```python
from build123d import *

# Parameters (mm, degrees)
F0_W     = 73.5
F0_H     = 5
F1_DEPTH = 10
F2_W     = 68.2
F2_H     = 5
F3_DEPTH = 8
F4_R     = 4
F5_DEPTH = 2
F6_W     = 5
F6_H     = 2
F7_DEPTH = 76.5
F8_R     = 3.99999
F9_DEPTH = 2.5
F10_R    = 4


# Not quite as in the source:
# - a fillet or chamfer is up to 0.001 mm smaller than in the source, because OpenCascade refuses the exact size


with BuildPart() as f1:
    # F0 (on Top) → F1 (new body)
    with BuildSketch(Plane.XY):
        Rectangle(F0_W, F0_H)
    extrude(amount=F1_DEPTH)

    # F2 (on face) → F3 (cut)
    with BuildSketch(Plane.XY.offset(10)):
        Rectangle(F2_W, F2_H)
    extrude(amount=-F3_DEPTH, mode=Mode.SUBTRACT)

    # F4
    f4_edges = [f1.edges().sort_by_distance(p)[0] for p in [
        (34.1, 0, 2),
        (-34.1, 0, 2),
    ]]
    fillet(f4_edges, radius=F4_R)

    # F5 (add): a face of the model
    f5_faces = [f1.faces().sort_by_distance(p)[0] for p in [
        (-35.425, 0, 10),
    ]]
    extrude(f5_faces, amount=F5_DEPTH)

    # F6 (on face) → F7 (join)
    with BuildSketch(Plane.YZ.offset(-34.1)):
        with Locations((0, 11)):
            Rectangle(F6_W, F6_H)
    extrude(amount=F7_DEPTH)

    # F8 (radius 4 in the source; OpenCascade refuses exactly that, so slightly less here)
    f8_edges = [f1.edges().sort_by_distance(p)[0] for p in [
        (-34.1, 0, 10),
        (34.1, 0, 10),
    ]]
    fillet(f8_edges, radius=F8_R)

    # F9 (cut): a face of the model
    f9_faces = [f1.faces().sort_by_distance(p)[0] for p in [
        (2.825, 0, 12),
    ]]
    extrude(f9_faces, amount=-F9_DEPTH, mode=Mode.SUBTRACT)

    # F10
    f10_edges = [f1.edges().sort_by_distance(p)[0] for p in [
        (36.75, 0, 0),
        (-36.75, 0, 9.5),
        (-36.75, 0, 0),
        (36.75, 0, 9.5),
    ]]
    fillet(f10_edges, radius=F10_R)


solid = f1.part
```
Input: part model. Units: mm. Frame: model coordinates. A direction names the side the tool comes from. Coordinates: 2 decimals unless noted, no trailing zeros. Loops run counter-clockwise (first coordinate to the right, second up) from the corner with the lowest first, then second, coordinate; pieces in that order, holes last. Notation, with made-up numbers: (-11, 81) -> (38, 81) arc R12 ccw to (38, 86) -> close; hole circle Ø5 at (39, 51). An arc over 180 degrees is marked (long way). Use a Markdown table: item, result.
1) Cut plane A-A (z = 8.25). Return the cut outline in (x, y), then the cut area to 3 significant figures.
Results found:
| item | result |
|---|---|
| outline | (-35.65, -2.5) -> (-33.41, -2.5) -> (-33.41, 2.5) -> (-35.65, 2.5) -> close; (33.41, -2.5) -> (35.65, -2.5) -> (35.65, 2.5) -> (33.41, 2.5) -> close |
| area | 22.5 mm2 |
2) Access query for faces 1 (the cylindrical face through (32.959, 0.035, 3.203)), 2 (the cylindrical face through (-35.547, 0.035, 1.141)), 3 (the flat face through (0, 0, 2)). Directions: +Z, -Z, +X, -X, +Y, -Y. A direction counts if a zero-diameter tool reaches every point of the face in a straight line with its end or side. Return the directions, or none.
Results found:
| item | result |
|---|---|
| face 1 | +Y, -Y |
| face 2 | -Z, -X, +Y, -Y |
| face 3 | +Z, +Y, -Y |
3) Cut plane C-C (x = 21.5). Return the cut outline in (y, z), then the cut area to 3 significant figures.
Results found:
| item | result |
|---|---|
| outline | (-2.5, 0) -> (2.5, 0) -> (2.5, 2) -> (-2.5, 2) -> close |
| area | 10.0 mm2 |
4) Pull-direction query (Z, two-part tool) for faces 4 (the flat face through (0, 0, 0)), 5 (the cylindrical face through (33.56, 0.04, 8.01)), 6 (the flat face through (-36.75, 0, 5)); classes: released by +Z, released by -Z, zero draft, split by the parting line, or undercut.
Results found:
| item | result |
|---|---|
| face 4 | released by -Z |
| face 5 | undercut |
| face 6 | zero draft |
5) Material intervals for line 1 along Z through (x, y) = (29, -1.35); line 2 along X through (y, z) = (0.9, 4); line 3 along Z through (x, y) = (-32.5, -2.2), sorted ascending. Write a range as from..to.
Results found:
| item | result |
|---|---|
| line 1 | z = 0..2 |
| line 2 | x = -36.75..-33.56, 33.56..36.75 |
| line 3 | z = 0..2.8, 9.2..9.5 |
6) Contact query for flat-ended pins moving along their axis: pin 1 (3 mm diameter, centred on x = 26, z = 3, fed in from +Y); pin 2 (2 mm diameter, centred on x = -21, y = 0, fed in from +Z). Output: stop coordinate, or through.
Results found:
| item | result |
|---|---|
| pin 1 | stops at y = 2.5 |
| pin 2 | stops at z = 2 |
